from build123d import *

# Parameters (mm, degrees)
F1_ANGLE = 30
F2_R     = 2
F3_R     = 2
F4_R     = 3
F5_DEPTH = 254.001


with BuildPart() as f1:
    # F0 (on Top) → F1 (revolve)
    with BuildSketch(Plane.XY):
        with BuildLine():
            Line((127, 194.31499), (127, 218.81499))
            ThreePointArc((127, 218.81499), (65.760199, 244.304311), (0, 253))
            Line((0, 253), (0, 246.65))
            ThreePointArc((0, 246.65), (62.544207, 238.588442), (121, 214.930739))
            Line((121, 214.930739), (121, 194.31499))
            Line((121, 194.31499), (127, 194.31499))
        make_face()
        with BuildLine():
            Line((0, 246.65), (0, 253))
            ThreePointArc((0, 253), (-65.760199, 244.304311), (-127, 218.81499))
            Line((-127, 218.81499), (-127, 194.31499))
            Line((-127, 194.31499), (-121, 194.31499))
            Line((-121, 194.31499), (-121, 214.930739))
            ThreePointArc((-121, 214.930739), (-62.544207, 238.588442), (0, 246.65))
        make_face()
    revolve(axis=Axis((69.665767, 0, 0), (1, 0, 0)), revolution_arc=F1_ANGLE)

    # F2
    f2_edges = [f1.edges().sort_by_distance(p)[0] for p in [
        (121, 207.607152, 55.628169),
    ]]
    fillet(f2_edges, radius=F2_R)

    # F3
    f3_edges = [f1.edges().sort_by_distance(p)[0] for p in [
        (-121, 207.607152, 55.628169),
    ]]
    fillet(f3_edges, radius=F3_R)

    # F4 (on face) → F5 (cut, through all)
    with BuildSketch(Plane(origin=(-127, 0, 0), x_dir=(0, -1, 0), z_dir=(-1, 0, 0))):
        with BuildLine():
            ThreePointArc((-199.78076, 23.037602), (-205.775963, 23.207197), (-199.799935, 22.698955))
            ThreePointArc((-199.799935, 22.698955), (-199.785558, 22.868008), (-199.78076, 23.037602))
        make_face()
        with BuildLine():
            ThreePointArc((-197.492142, 38.12701), (-203.478908, 38.40848), (-197.544959, 37.566552))
            ThreePointArc((-197.544959, 37.566552), (-197.505375, 37.845539), (-197.492142, 38.12701))
        make_face()
        with BuildLine():
            ThreePointArc((-200.938163, 7.689393), (-200.936833, 7.724924), (-200.935924, 7.760468))
            ThreePointArc((-200.935924, 7.760468), (-200.935491, 7.789912), (-200.935346, 7.819359))
            ThreePointArc((-200.935346, 7.819359), (-203.888144, 10.818988), (-206.933861, 7.913752))
            Line((-206.933861, 7.913752), (-200.938163, 7.689393))
        make_face()
        with BuildLine():
            ThreePointArc((-206.933861, 7.913752), (-204.047527, 4.821457), (-200.938163, 7.689393))
            Line((-200.938163, 7.689393), (-206.933861, 7.913752))
        make_face()
        with Locations((-203.949443, -7.442613)):
            Circle(F4_R)
        with Locations((-202.822972, -22.662963)):
            Circle(F4_R)
        with Locations((-200.562232, -37.756572)):
            Circle(F4_R)
        with Locations((-197.179868, -52.639032)):
            Circle(F4_R)
        with Locations((-192.694793, -67.227112)):
            Circle(F4_R)
        with Locations((-187.132091, -81.439231)):
            Circle(F4_R)
        with Locations((-180.52287, -95.195909)):
            Circle(F4_R)
        with Locations((-172.904092, -108.420213)):
            Circle(F4_R)
        with Locations((-164.318365, -121.038187)):
            Circle(F4_R)
        with Locations((-154.813702, -132.979267)):
            Circle(F4_R)
        with Locations((-144.443259, -144.176672)):
            Circle(F4_R)
        with Locations((-133.26503, -154.567783)):
            Circle(F4_R)
        with Locations((-121.341529, -164.094489)):
            Circle(F4_R)
        with Locations((-108.739437, -172.703511)):
            Circle(F4_R)
        with Locations((-95.52923, -180.346705)):
            Circle(F4_R)
        with Locations((-81.784784, -186.981328)):
            Circle(F4_R)
        with Locations((-67.582966, -192.570274)):
            Circle(F4_R)
        with Locations((-53.003195, -197.08229)):
            Circle(F4_R)
        with Locations((-38.12701, -200.492142)):
            Circle(F4_R)
        with Locations((-23.037602, -202.78076)):
            Circle(F4_R)
        with Locations((-7.819359, -203.935346)):
            Circle(F4_R)
        with Locations((7.442613, -203.949443)):
            Circle(F4_R)
        with Locations((22.662963, -202.822972)):
            Circle(F4_R)
        with Locations((37.756572, -200.562232)):
            Circle(F4_R)
        with Locations((52.639032, -197.179868)):
            Circle(F4_R)
        with Locations((67.227112, -192.694793)):
            Circle(F4_R)
        with Locations((81.439231, -187.132091)):
            Circle(F4_R)
        with Locations((95.195909, -180.52287)):
            Circle(F4_R)
        with Locations((108.420213, -172.904092)):
            Circle(F4_R)
        with Locations((121.038187, -164.318365)):
            Circle(F4_R)
        with Locations((132.979267, -154.813702)):
            Circle(F4_R)
        with Locations((144.176672, -144.443259)):
            Circle(F4_R)
        with Locations((154.567783, -133.26503)):
            Circle(F4_R)
        with Locations((164.094489, -121.341529)):
            Circle(F4_R)
        with Locations((172.703511, -108.739437)):
            Circle(F4_R)
        with Locations((180.346705, -95.52923)):
            Circle(F4_R)
        with Locations((186.981328, -81.784784)):
            Circle(F4_R)
        with Locations((192.570274, -67.582966)):
            Circle(F4_R)
        with Locations((197.08229, -53.003195)):
            Circle(F4_R)
        with Locations((200.492142, -38.12701)):
            Circle(F4_R)
        with Locations((202.78076, -23.037602)):
            Circle(F4_R)
        with Locations((203.935346, -7.819359)):
            Circle(F4_R)
        with Locations((203.949443, 7.442613)):
            Circle(F4_R)
        with Locations((202.822972, 22.662963)):
            Circle(F4_R)
        with Locations((200.562232, 37.756572)):
            Circle(F4_R)
        with Locations((197.179868, 52.639032)):
            Circle(F4_R)
        with Locations((192.694793, 67.227112)):
            Circle(F4_R)
        with Locations((187.132091, 81.439231)):
            Circle(F4_R)
        with Locations((180.52287, 95.195909)):
            Circle(F4_R)
        with Locations((172.904092, 108.420213)):
            Circle(F4_R)
        with Locations((164.318365, 121.038187)):
            Circle(F4_R)
        with Locations((154.813702, 132.979267)):
            Circle(F4_R)
        with Locations((144.443259, 144.176672)):
            Circle(F4_R)
        with Locations((133.26503, 154.567783)):
            Circle(F4_R)
        with Locations((121.341529, 164.094489)):
            Circle(F4_R)
        with Locations((108.739437, 172.703511)):
            Circle(F4_R)
        with Locations((95.52923, 180.346705)):
            Circle(F4_R)
        with Locations((81.784784, 186.981328)):
            Circle(F4_R)
        with Locations((67.582966, 192.570274)):
            Circle(F4_R)
        with Locations((53.003195, 197.08229)):
            Circle(F4_R)
        with Locations((38.12701, 200.492142)):
            Circle(F4_R)
        with Locations((23.037602, 202.78076)):
            Circle(F4_R)
        with Locations((7.819359, 203.935346)):
            Circle(F4_R)
        with Locations((-7.442613, 203.949443)):
            Circle(F4_R)
        with Locations((-22.662963, 202.822972)):
            Circle(F4_R)
        with Locations((-37.756572, 200.562232)):
            Circle(F4_R)
        with Locations((-52.639032, 197.179868)):
            Circle(F4_R)
        with Locations((-67.227112, 192.694793)):
            Circle(F4_R)
        with Locations((-81.439231, 187.132091)):
            Circle(F4_R)
        with Locations((-95.195909, 180.52287)):
            Circle(F4_R)
        with Locations((-108.420213, 172.904092)):
            Circle(F4_R)
        with Locations((-121.038187, 164.318365)):
            Circle(F4_R)
        with Locations((-132.979267, 154.813702)):
            Circle(F4_R)
        with Locations((-144.176672, 144.443259)):
            Circle(F4_R)
        with Locations((-154.567783, 133.26503)):
            Circle(F4_R)
        with Locations((-164.094489, 121.341529)):
            Circle(F4_R)
        with Locations((-172.703511, 108.739437)):
            Circle(F4_R)
        with Locations((-180.346705, 95.52923)):
            Circle(F4_R)
        with Locations((-186.981328, 81.784784)):
            Circle(F4_R)
        with Locations((-192.570274, 67.582966)):
            Circle(F4_R)
        with Locations((-197.08229, 53.003195)):
            Circle(F4_R)
    extrude(amount=-F5_DEPTH, mode=Mode.SUBTRACT)


solid = f1.part
Geometry: final body of the model. Coordinates: model frame, mm. A direction names the side the tool comes from. Coordinates: 2 decimals unless noted, no trailing zeros. One line per question, with ' | ' between items. Start each with the question number.
Item 1: Pin query (flat end, axial travel): pin 1 Ø3 at (x, z) = (-18.5, 97) entering from -Y; pin 2 Ø1.5 at (x, z) = (-88.5, 73) entering from +Y; pin 3 Ø5 at (x, z) = (36, 93.5) entering from +Y. Return the tip coordinate at first contact, or that it passes through.
Item 2: Draft query along Y for faces 3 (the flat face through (-10, 214.517, 123.852)), 4 (the flat face through (-10, 248, 0)), 5 (the cylindrical face through (-124.04, 200.08, 53.14)). Return one class per face: released by +Y, released by -Y, zero draft, split by the parting line, or undercut.
Item 3: Ray query, probe 1 along X at (y, z) = (203, 41); probe 2 along X at (y, z) = (189.5, 101.5); probe 3 along Y at (x, z) = (45.5, 50). Return the intervals inside material, ascending. Write a range as [from, to].
Item 4: Set-up query: faces 1 (the cylindrical face through (-124.042, 192.961, 70.557)), 2 (the flat face through (-121, 191, 54)). Return all of +Z, -Z, +X, -X, +Y, -Y with unobstructed straight access to the full face (end or side cutting, diameter ignored); none if empty.
A:
1) pin 1: stops at y = 225.36 | pin 2: stops at y = 225.87 | pin 3: stops at y = 233.38
2) face 3: released by -Y | face 4: zero draft | face 5: undercut
3) probe 1: x = [-127, -121], [121, 127] | probe 2: x = [-127, -120.59], [120.59, 127] | probe 3: y = [237.2, 243.8]
4) face 1: +X, -X | face 2: -Z, -Y
